Model file for the job. Use its own axes, mm. Face numbers are marked on the shaded views. Coordinates: 2 decimals unless noted, no trailing zeros. Order: outer loops, then holes, each group sorted by start corner. A loop starts at its lowest first (then second) coordinate and runs counter-clockwise, first axis right, second up.
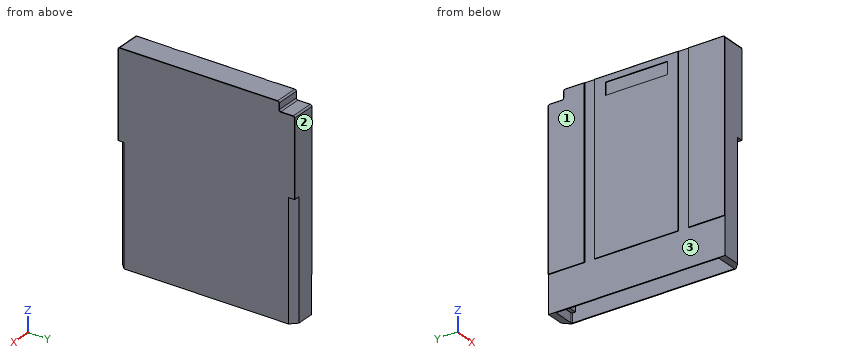
from build123d import *

# Parameters (mm, degrees)
F1_DEPTH  = 3.875
F3_DEPTH  = 38
F4_W      = 27
F4_H      = 54
F4_W_2    = 20
F4_H_2    = 4
F4_W_3    = 11.7
F5_DEPTH  = 0.25
F8_R      = 0.5
F9_R      = 0.1
F11_W     = 7.15
F11_H     = 50
F12_DEPTH = 62
F14_DEPTH = 3


# Not quite as in the source:
# - a pattern or mirror of a feature is missing from the dataset's text; its kind, count and spacing are read off the source's solid


with BuildPart() as f1:
    # F0 (on Right) → F1 (new body, symmetric)
    with BuildSketch(Plane.YZ):
        Polygon((23.5, 33), (-28.5, 33), (-28.5, -33), (28.5, -33), (28.5, 30), (23.5, 30), align=None)
    extrude(amount=F1_DEPTH, both=True)

    # F2 (on face) → F3 (cut)
    with BuildSketch(Plane(origin=(0, 0, -33), x_dir=(1, 0, 0), z_dir=(0, 0, -1))):
        Polygon((3.875, 28.5), (1.875, 28.5), (3.875, 26.5), align=None)
        Polygon((3.875, -26.5), (1.875, -28.5), (3.875, -28.5), align=None)
    extrude(amount=-F3_DEPTH, mode=Mode.SUBTRACT)

    # F4 (on face) → F5 (join)
    with BuildSketch(Plane(origin=(-3.875, 0, 0), x_dir=(0, -1, 0), z_dir=(-1, 0, 0))):
        with Locations((0, 6)):
            Rectangle(F4_W, F4_H)
        with Locations((0, 29)):
            Rectangle(F4_W_2, F4_H_2, mode=Mode.SUBTRACT)
        with Locations((22.65, 6)):
            Rectangle(F4_W_3, F4_H)
        Polygon((-28.5, 30), (-28.5, -21), (-16.8, -21), (-16.8, 33), (-23.5, 33), (-23.5, 30), align=None)
    extrude(amount=F5_DEPTH)

    # F8
    f8_edges = [f1.edges().sort_by_distance(p)[0] for p in [
        (-0.125, 23.5, 33),
        (-0.125, 23.5, 30),
        (-0.125, 28.5, 30),
        (-0.125, -28.5, 33),
    ]]
    fillet(f8_edges, radius=F8_R)

    # F9
    f9_edges = [f1.edges().sort_by_distance(p)[0] for p in [
        (3.875, -2.5, 33),
        (3.875, 26, 30),
        (-4.125, 26, 30),
        (-4.125, 23.5, 31.5),
        (3.875, 23.5, 31.5),
        (-4.125, 19.9, 33),
        (-4.125, 0, 33),
        (-4.125, -22.4, 33),
        (-4.125, -28.5, 5.75),
        (3.875, -28.5, 18.75),
        (-4.125, 28.5, 4.25),
        (-4.125, -28.353553, 32.853553),
        (3.875, -28.353553, 32.853553),
        (3.875, 23.646447, 30.146447),
        (3.875, 23.353553, 32.853553),
        (3.875, 28.353553, 29.853553),
        (3.875, 28.5, 17.25),
        (-4.125, 23.353553, 32.853553),
        (-4.125, 28.353553, 29.853553),
        (-4.125, 23.646447, 30.146447),
    ]]
    fillet(f9_edges, radius=F9_R)

    # F11 (on face) → F12 (cut)
    with BuildSketch(Plane(origin=(0, 0, -33), x_dir=(1, 0, 0), z_dir=(0, 0, -1))):
        Rectangle(F11_W, F11_H)
    extrude(amount=-F12_DEPTH, mode=Mode.SUBTRACT)

    # F13 (on face) → F14 (cut)
    with BuildSketch(Plane(origin=(0, 0, -33), x_dir=(1, 0, 0), z_dir=(0, 0, -1))):
        with BuildLine():
            Line((3.575, -25), (-3.575, -25))
            Line((-3.575, -25), (-3.575, -26))
            ThreePointArc((-3.575, -26), (-3.5017766953, -26.1767766953), (-3.325, -26.25))
            Line((-3.325, -26.25), (3.325, -26.25))
            ThreePointArc((3.325, -26.25), (3.5017766953, -26.1767766953), (3.575, -26))
            Line((3.575, -26), (3.575, -25))
        make_face()
    f14 = extrude(amount=-F14_DEPTH, mode=Mode.SUBTRACT)

    # F14_copies: F14 across plane
    add(f14.mirror(Plane(origin=(0, 0, 0), x_dir=(0, 0, -1), z_dir=(0, -1, 0))), mode=Mode.SUBTRACT)


solid = f1.part
Q1. Cut at A-A, the plane z = 23.5. List the corners of the cut face in (x, y) (3 decimals), plus the area to 3 significant figures.
Established:
outline: (-4.125, -28.4) arc R0.1 ccw to (-4.025, -28.5) - (3.775, -28.5) arc R0.1 ccw to (3.875, -28.4) - (3.875, 28.4) arc R0.1 ccw to (3.775, 28.5) - (-4.025, 28.5) arc R0.1 ccw to (-4.125, 28.4) - (-4.125, 16.8) - (-3.875, 16.8) - (-3.875, 13.5) - (-4.125, 13.5) - (-4.125, -13.5) - (-3.875, -13.5) - (-3.875, -16.8) - (-4.125, -16.8) - close; hole (-3.575, -25) - (3.575, -25) - (3.575, 25) - (-3.575, 25) - close
area: 96.8 mm2
Q2. Mould opens along Y. For the marked faces 1, 2 and 3 say: pulls with the +Y half, pulls with the -Y half, needs draft (parallel to the pull), parting line crosses it, or undercut.
Established:
face 1: needs draft
face 2: pulls with the +Y half
face 3: undercut
Q3. Probe line 1 (X direction, y = 11.5, z = -7.5) (3 decimals); line 2 (X direction, y = 16, z = 8) (3 decimals); line 3 (Y direction, x = -2, z = -18.5). List the from-to ranges inside material, lowest first.
Established:
line 1: x = -4.125 to -3.575, 3.575 to 3.875
line 2: x = -3.875 to -3.575, 3.575 to 3.875
line 3: y = -28.5 to -25, 25 to 28.5
Q4. Cut at B-B, the plane y = 7. List the corners of the cut face in (x, z) (3 decimals), plus the area to 3 significant figures.
Established:
outline: (-4.125, -21) - (-3.875, -21) - (-3.875, -33) - (-3.575, -33) - (-3.575, 29) - (3.575, 29) - (3.575, -33) - (3.875, -33) - (3.875, 32.9) arc R0.1 ccw to (3.775, 33) - (-4.025, 33) arc R0.1 ccw to (-4.125, 32.9) - (-4.125, 31) - (-3.875, 31) - (-3.875, 27) - (-4.125, 27) - close
area: 80.7 mm2
Q5. Drop flat-ended pins along their axis: P1, Ø0.6, axis at x = 3, y = 28, coming from the -Z side; P2, Ø1.2, axis at y = -2.5, z = 28.5, coming from the -X side (3 decimals); P3, Ø4, axis at x = 1.5, y = -6, coming from the -Z side. Give the stop position or say it passes through.
Established:
P1: stops at z = 5
P2: stops at x = -3.875
P3: stops at z = 29
Q6. Cut at D-D, the plane z = -7. List the corners of the cut face in (x, y) (3 decimals), plus the area to 3 significant figures.
Established:
outline: (-4.125, -28.4) arc R0.1 ccw to (-4.025, -28.5) - (1.875, -28.5) - (3.875, -26.5) - (3.875, 26.5) - (1.875, 28.5) - (-4.025, 28.5) arc R0.1 ccw to (-4.125, 28.4) - (-4.125, 16.8) - (-3.875, 16.8) - (-3.875, 13.5) - (-4.125, 13.5) - (-4.125, -13.5) - (-3.875, -13.5) - (-3.875, -16.8) - (-4.125, -16.8) - close; hole (-3.575, -25) - (3.575, -25) - (3.575, 25) - (-3.575, 25) - close
area: 92.8 mm2
Q7. Cut at C-C, the plane x = -0.5. List the corners of the cut face in (y, z).
Established:
outline: (-28.5, -33) - (-26.25, -33) - (-26.25, -30) - (-25, -30) - (-25, 29) - (25, 29) - (25, -30) - (26.25, -30) - (26.25, -33) - (28.5, -33) - (28.5, 29.5) arc R0.5 ccw to (28, 30) - (24, 30) arc R0.5 cw to (23.5, 30.5) - (23.5, 32.5) arc R0.5 ccw to (23, 33) - (-28, 33) arc R0.5 ccw to (-28.5, 32.5) - close
